from build123d import *

# Parameters (mm, degrees)
SKETCH031_W             = 40
SKETCH031_H             = 18
SKETCH031_R             = 1.05
PAD019_DEPTH            = 1.2
SKETCH032_R             = 7.95
PAD020_DEPTH            = 12.2
SKETCH033_W             = 10
SKETCH033_H             = 9
PAD021_DEPTH            = 3.96
BODY005_PLACEMENT_ANGLE = 90


with BuildPart() as part:
    # Sketch031 → Pad019 (new body)
    with BuildSketch(Plane.XZ):
        Rectangle(SKETCH031_W, SKETCH031_H)
        with Locations((-18.75, 7.75)):
            Circle(SKETCH031_R, mode=Mode.SUBTRACT)
        with Locations((-18.75, -7.75)):
            Circle(SKETCH031_R, mode=Mode.SUBTRACT)
        with Locations((18.75, -7.75)):
            Circle(SKETCH031_R, mode=Mode.SUBTRACT)
        with Locations((18.75, 7.75)):
            Circle(SKETCH031_R, mode=Mode.SUBTRACT)
    extrude(amount=PAD019_DEPTH)

    # Sketch032 (on Face10 of Pad019) → Pad020 (join)
    with BuildSketch(Plane.XZ.offset(1.2)):
        with Locations((-10.825, 0)):
            Circle(SKETCH032_R)
        with Locations((10.825, 0)):
            Circle(SKETCH032_R)
    extrude(amount=PAD020_DEPTH)

    # Sketch033 (on Face4 of Pad020) → Pad021 (join)
    with BuildSketch(Plane(origin=(0, 0, 0), x_dir=(1, 0, 0), z_dir=(0, 1, 0))):
        with Locations((0, -11)):
            Rectangle(SKETCH033_W, SKETCH033_H)
    extrude(amount=PAD021_DEPTH)


with BuildPart() as part_1:
    # Body005 placement: moved
    add(part.part.moved(Location((43, 0, 53))).rotate(Axis((43, 0, 53), (0, 0, 1)), BODY005_PLACEMENT_ANGLE))


solid = part_1.part
Model file for the job. Use its own axes, mm. A direction names the side the tool comes from. Give positions to 0.01 mm unless a question says otherwise; leave off trailing zeros. Loops run counter-clockwise (first coordinate to the right, second up) from the corner with the lowest first, then second, coordinate; pieces in that order, holes last. Notation, with made-up numbers: (4, -12) -> (55, -12) arc R9 cw to (55, -7) -> close; hole circle Ø4 at (42.5, 57.25). An arc over 180 degrees is marked (long way). Use a Markdown table: item, result. Add a question column.
(1) Tool access for faces 1 (the flat face through (44, 0, 62)), 2 (the flat face through (41, -5, 64)), 3 (the flat face through (41, 0, 59.5)), 4 (the flat face through (44.2, 0, 53)): list every direction of +Z, -Z, +X, -X, +Y, -Y with a clear straight run to the whole face (end or side of a thin tool).
(2) Slice it at C-C on y = 15.5. List the corners of the cut face in (x, z).
(3) Drop flat-ended pins along their axis: pin 1 Ø3 at (x, z) = (40.5, 62.5) entering from -Y; pin 2 Ø2 at (y, z) = (-9.5, 52) entering from -X; pin 3 Ø3.5 at (y, z) = (-18.75, 45.25) entering from +X. Give the stop position or say it passes through.
(4) Wall check: line 1 along Z through (x, y) = (43.85, 18.75); line 2 along X through (y, z) = (1, 48.5); line 3 along X through (y, z) = (-4, 60.75). Give the ranges that are in metal, low to high.
(5) Slice it at A-A on x = 43.75. List the corners of the cut face in (y, z), and give its area (3 significant figures).
(6) Slice it at B-B on z = 53. List the corners of the cut face in (x, y) (3 decimals), and give its area (3 significant figures).
(7) Slice it at D-D on z = 46.75. List the corners of the cut face in (x, y), and give its area (3 significant figures).
Filled sheet:
| question | item | result |
|---|---|---|
| 1 | face 1 | +Z, +X, +Y, -Y |
| 1 | face 2 | +Z, -Z, -X, -Y |
| 1 | face 3 | -Z, -X, +Y, -Y |
| 1 | face 4 | +X |
| 2 | outline | (43, 44) -> (44.2, 44) -> (44.2, 46.57) -> (56.4, 46.57) -> (56.4, 59.43) -> (44.2, 59.43) -> (44.2, 62) -> (43, 62) -> close |
| 3 | pin 1 | y = -5 |
| 3 | pin 2 | x = 43 |
| 3 | pin 3 | x = 44.2 |
| 4 | line 1 | 44 to 44.2, 46.3 to 59.7, 61.8 to 62 |
| 4 | line 2 | 43 to 44.2 |
| 4 | line 3 | 39.04 to 44.2 |
| 5 | outline | (-20, 44) -> (20, 44) -> (20, 62) -> (-20, 62) -> close; hole circle Ø2.1 at (-18.75, 45.25); hole circle Ø2.1 at (-18.75, 60.75); hole circle Ø2.1 at (18.75, 45.25); hole circle Ø2.1 at (18.75, 60.75) |
| 5 | area | 706 mm2 |
| 6 | outline | (43, -20) -> (44.2, -20) -> (44.2, -18.775) -> (56.4, -18.775) -> (56.4, -2.875) -> (44.2, -2.875) -> (44.2, 2.875) -> (56.4, 2.875) -> (56.4, 18.775) -> (44.2, 18.775) -> (44.2, 20) -> (43, 20) -> close |
| 6 | area | 436 mm2 |
| 7 | outline | (43, -20) -> (44.2, -20) -> (44.2, -15.74) -> (56.4, -15.74) -> (56.4, -5.91) -> (44.2, -5.91) -> (44.2, 5.91) -> (56.4, 5.91) -> (56.4, 15.74) -> (44.2, 15.74) -> (44.2, 20) -> (43, 20) -> close |
| 7 | area | 288 mm2 |
